Part model, mm, in its own coordinate system. A direction names the side the tool comes from. Round coordinates to 2 decimals unless told otherwise and drop trailing zeros. Write each loop counter-clockwise with the first axis right and the second up, starting at its lowest first coordinate (ties: lowest second). Pieces come first, ordered by that corner, then holes. Notation, with made-up numbers: M 35,-24 L 80,-24 A12 cw 80,-10 Z; hole C 53,55 d8. An arc over 180 degrees is marked long. Use a Markdown table: item, result. Add a question column.
1) Slice it at A-A on z = -144. Write the cut outline in (x, y), plus the area to 3 significant figures.
2) Slice it at B-B on x = -104.5. Write the cut outline in (y, z), plus the area to 3 significant figures.
3) Two-plate mould, pull along Y, no slides. Class faces 1 (the face through (-61, 94, -181)), 2 (the face through (-61, 91, -185)), 3 (the face through (-61, 185, -91)): released by +Y, released by -Y, zero draft, split by the parting line, or undercut.
4) Wall check: probe 1 along Y at (x, z) = (-44, -152); probe 2 along X at (y, z) = (137, -60.5); probe 3 along Y at (x, z) = (-33, -75). Give the ranges that are in metal, low to high.
5) Which spindle directions (+Z, -Z, +X, -X, +Y, -Y) get a long thin tool onto all of the face, cutting with end or side? Do faces 4 (the face through (-117.972, 91.261, -68.445)), 5 (the face through (-61, 4, -158)). Say none if no direction does.
6) Drop flat-ended pins along their axis: P1, Ø2, axis at x = -56.5, y = 2.5, coming from the +Z side; P2, Ø3, axis at x = -37, z = -47.5, coming from the -Y side. Give the stop position or say it passes through.
7) Slice it at C-C on z = -36. Write the cut outline in (x, y).
```python
from build123d import *

# Parameters (mm, degrees)
F0_W     = 120
F0_H     = 185
F1_DEPTH = 185
F3_DEPTH = 120
F4_W     = 112
F4_H     = 177
F5_DEPTH = 181


with BuildPart() as f1:
    # F0 (on Front) → F1 (new body)
    with BuildSketch(Plane.XZ):
        with Locations((-60, -92.5)):
            Rectangle(F0_W, F0_H)
    extrude(amount=-F1_DEPTH)

    # F2 (on face) → F3 (cut, through all)
    with BuildSketch(Plane.YZ):
        Polygon((4, -135), (181, 0), (0, 0), (0, -135), align=None)
    extrude(amount=-F3_DEPTH, mode=Mode.SUBTRACT)

    # F4 (on Top) → F5 (cut)
    with BuildSketch(Plane.XY):
        with Locations((-60, 92.5)):
            Rectangle(F4_W, F4_H)
    extrude(amount=-F5_DEPTH, mode=Mode.SUBTRACT)


solid = f1.part
```
Entries:
| question | item | result |
|---|---|---|
| 1 | outline | M -120,0 L 0,0 L 0,185 L -120,185 Z; hole M -116,4 L -4,4 L -4,181 L -116,181 Z |
| 1 | area | 2,380 mm^2 |
| 2 | outline | M 0,-185 L 185,-185 L 185,0 L 181,0 L 181,-181 L 4,-181 L 4,-135 L 0,-135 Z |
| 2 | area | 1,650 mm^2 |
| 3 | face 1 | undercut |
| 3 | face 2 | zero draft |
| 3 | face 3 | released by +Y |
| 4 | probe 1 | y = 0 to 4, 181 to 185 |
| 4 | probe 2 | x = -120 to -116, -4 to 0 |
| 4 | probe 3 | y = 181 to 185 |
| 5 | face 4 | +Z, +X, -X, -Y |
| 5 | face 5 | +Z |
| 6 | P1 | stops at z = -135 |
| 6 | P2 | stops at y = 181 |
| 7 | outline | M -120,133.8 L -116,133.8 L -116,181 L -4,181 L -4,133.8 L 0,133.8 L 0,185 L -120,185 Z |
